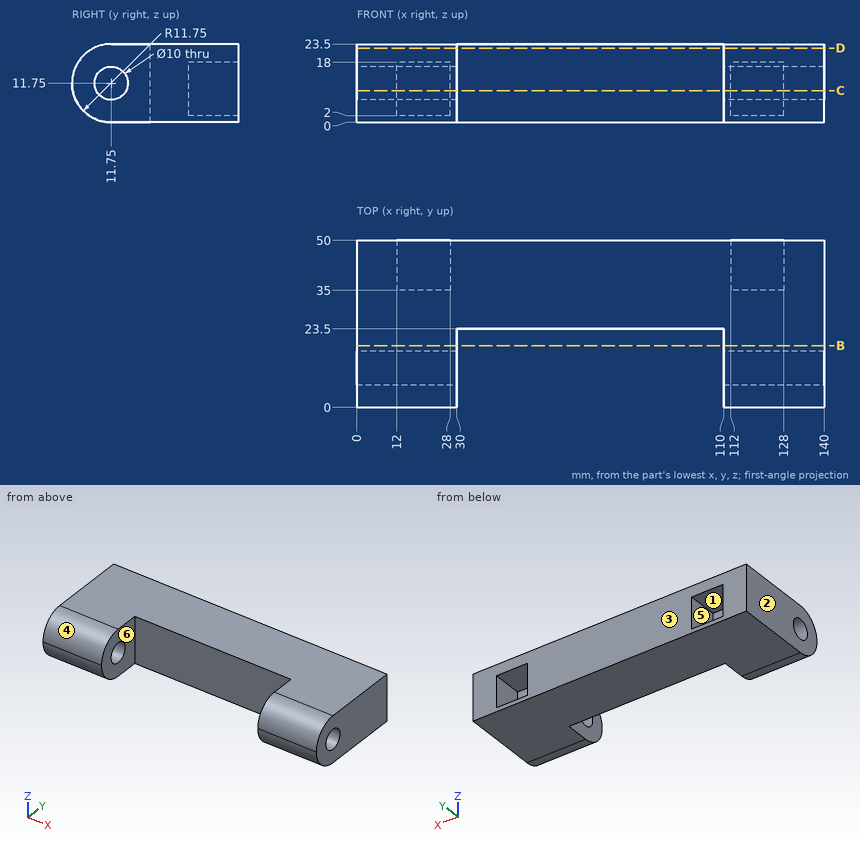
Design review of the part shown in the three views and the two pictorial views. Dimensions are in mm from the part's minimum x, y and z. A direction names the side the tool comes from. Coordinates: 2 decimals unless noted, no trailing zeros. Order: outer loops, then holes, each group sorted by start corner. A loop starts at its lowest first (then second) coordinate and runs counter-clockwise, first axis right, second up. Notation, with made-up numbers: (48, -4) - (53, -4) arc R19 cw to (53, 23) - close; hole circle Ø2 at (68, 21.25). An arc over 180 degrees is marked (long way). Answer as CSV lines item,"result". Start each with the question number.
1) Add section C-C (z = 9.5). State the section outline as (x, y) points, then the cut area to 3 significant figures.
2) Draft analysis for pull direction X (two halves, no side actions). For the marked faces 1, 2 and 3, state which applies: +X half, -X half, draft (parallel to the pull), parting line (faces both ways), or undercut.
3) Add section D-D (z = 22.25). State the section outline as (x, y) points.
4) Machinability: for the marked faces 4, 5 and 6, which of the approach directions +Z, -Z, +X, -X, +Y, -Y give a long, thin tool a straight path to every point of the face, cutting with its end or side? Answer none if there is none.
5) Add section B-B (y = 18.5). State the section outline as (x, z) points, then the cut area to 3 significant figures.
6) Insertion check: P1, Ø7.5, axis at y = 43.5, z = 10, coming from the -X side; P2, Ø7, axis at x = 90, z = 9.5, coming from the -Y side; P3, Ø5, axis at x = 124, z = 7, coming from the +Y side. Each pin has a flat end and moves straight along its axis. Give the tip position at first contact, or say it passes through.
7) To check wall thickness, follow line 1 along X through (y, z) = (36.5, 7.75); line 2 along X through (y, z) = (13.5, 5.25); line 3 along Z through (x, y) = (16.75, 11.75). State the ranges of each line that lie inside material, in increasing order. Write a range as [from, to].
Result:
1,outline,"(0, 0.22) - (30, 0.22) - (30, 7.28) - (0, 7.28) - close; (0, 16.22) - (30, 16.22) - (30, 23.5) - (110, 23.5) - (110, 16.22) - (140, 16.22) - (140, 50) - (128, 50) - (128, 35) - (112, 35) - (112, 50) - (28, 50) - (28, 35) - (12, 35) - (12, 50) - (0, 50) - close; (110, 0.22) - (140, 0.22) - (140, 7.28) - (110, 7.28) - close"
1,area,"4,090 mm^2"
2,face 1,"undercut"
2,face 2,"-X half"
2,face 3,"draft"
3,outline,"(0, 6.48) - (30, 6.48) - (30, 23.5) - (110, 23.5) - (110, 6.48) - (140, 6.48) - (140, 50) - (0, 50) - close"
4,face 4,"+Z, +X, -X, -Y"
4,face 5,"+Y"
4,face 6,"+Z, -Z, -Y"
5,outline,"(0, 0) - (30, 0) - (30, 23.5) - (0, 23.5) - close; (110, 0) - (140, 0) - (140, 23.5) - (110, 23.5) - close"
5,area,"1,410 mm^2"
6,P1,"x = 0"
6,P2,"y = 23.5"
6,P3,"y = 35"
7,line 1,"[0, 12], [28, 112], [128, 140]"
7,line 2,"[0, 30], [110, 140]"
7,line 3,"[0, 6.75], [16.75, 23.5]"
